Work out the finished part from the listing and answer in its coordinate system (mm). A direction names the side the tool comes from. Give positions to 0.01 mm unless a question says otherwise; leave off trailing zeros. Order: outer loops, then holes, each group sorted by start corner. A loop starts at its lowest first (then second) coordinate and runs counter-clockwise, first axis right, second up. Notation, with made-up numbers: (-30.75, 6) -> (-24.75, 6) arc R17 ccw to (-24.75, 15) -> close; hole circle Ø2 at (-39, 57.5). An arc over 180 degrees is marked (long way). Use a Markdown table: item, result. Add a question column.
```python
from build123d import *

# Parameters (mm, degrees)
EXTRUDE_1_DEPTH     = 18
CUT_EXTRUDE_1_DEPTH = 16
HOLE_WIZARD_M51_D   = 5.5
HOLE_WIZARD_M52_D   = 5.5


with BuildPart() as part:
    # Эскиз1 → Бобышка-Вытянуть1 (new body)
    with BuildSketch(Plane.XY):
        Polygon((0, 0), (0, 8), (30.5, 38.5), (38.5, 38.5), (38.5, 0), align=None)
    extrude(amount=EXTRUDE_1_DEPTH)

    # Эскиз2 → Вырез-Вытянуть1 (cut)
    with BuildSketch(Plane.XY.offset(18)):
        Polygon((0, 2), (36.5, 2), (36.5, 38.5), (30.5, 38.5), (0, 8), align=None)
    extrude(amount=-CUT_EXTRUDE_1_DEPTH, mode=Mode.SUBTRACT)

    # Отверстие с зазором M51 (through all)
    with Locations(Plane(origin=(0, 2, 0), x_dir=(1, 0, 0), z_dir=(0, 1, 0))):
        with Locations((8.5, -9), (28.5, -9)):
            Hole(HOLE_WIZARD_M51_D / 2)

    # Отверстие с зазором M52 (through all)
    with Locations(Plane.ZY.offset(-36.5)):
        with Locations((9, 10), (9, 30)):
            Hole(HOLE_WIZARD_M52_D / 2)


solid = part.part
```
1) The part is cut by section A-A, the plane y = 30. Determine the outline of the cut face in (x, z), then the cut area to 3 significant figures.
2) The part is cut by section D-D, the plane y = 16.5. Determine the outline of the cut face in (x, z), then the cut area to 3 significant figures.
3) Determine the mould class of faces 1 (the flat face through (15, 23, 1)), 2 (the cylindrical face through (37.51, 32.32, 7.52)), 3 (the flat face through (38.5, 20, 9)), 4 (the cylindrical face through (31.247, 0.986, 8.879)) for opening direction X: released by +X, released by -X, zero draft, split by the parting line, or undercut.
4) Straight lines are drawn through the part: line 1 (Y direction, x = 37, z = 9); line 2 (X direction, y = 1.4, z = 9); line 3 (Z direction, x = 8.5, y = 0.9). For each, find the intervals that lie inside material, in ascending order.
5) Which of the six approach directions +Z, -Z, +X, -X, +Y, -Y give full straight-line access (tool end or side, diameter ignored) to faces 5 (the cylindrical face through (37.51, 12.32, 7.52)), 6 (the flat face through (18, 2, 10))?
6) The part is cut by section C-C, the plane x = 28.5. Determine the outline of the cut face in (y, z), then the cut area to 3 significant figures.
7) The part is cut by section B-B, the plane z = 9. Determine the outline of the cut face in (x, y).
8) Flat-ended cylindrical pins translate along their axes: pin 1 (10 mm diameter, centred on x = 11.5, y = 10, fed in from +Z); pin 2 (1 mm diameter, centred on y = 34.5, z = 12, fed in from -X); pin 3 (5 mm diameter, centred on x = 28.5, z = 9, fed in from -Y); pin 4 (1.5 mm diameter, centred on x = 15.5, z = 4.5, fed in from +Y). Find the tip coordinate at first contact, or state that the pin passes through.
A:
| question | item | result |
|---|---|---|
| 1 | outline | (22, 0) -> (38.5, 0) -> (38.5, 6.25) -> (36.5, 6.25) -> (36.5, 2) -> (22, 2) -> close; (36.5, 11.75) -> (38.5, 11.75) -> (38.5, 18) -> (36.5, 18) -> close |
| 1 | area | 54.0 mm^2 |
| 2 | outline | (8.5, 0) -> (38.5, 0) -> (38.5, 18) -> (36.5, 18) -> (36.5, 2) -> (8.5, 2) -> close |
| 2 | area | 92.0 mm^2 |
| 3 | face 1 | released by -X |
| 3 | face 2 | zero draft |
| 3 | face 3 | released by +X |
| 3 | face 4 | undercut |
| 4 | line 1 | 0 to 7.25, 12.75 to 27.25, 32.75 to 38.5 |
| 4 | line 2 | 0 to 5.75, 11.25 to 25.75, 31.25 to 38.5 |
| 4 | line 3 | 0 to 6.25, 11.75 to 18 |
| 5 | face 5 | +X, -X |
| 5 | face 6 | +Z, -X, +Y |
| 6 | outline | (0, 0) -> (36.5, 0) -> (36.5, 2) -> (2, 2) -> (2, 6.25) -> (0, 6.25) -> close; (0, 11.75) -> (2, 11.75) -> (2, 18) -> (0, 18) -> close |
| 6 | area | 94.0 mm^2 |
| 7 | outline | (0, 0) -> (5.75, 0) -> (5.75, 2) -> (0, 2) -> close; (11.25, 0) -> (25.75, 0) -> (25.75, 2) -> (11.25, 2) -> close; (31.25, 0) -> (38.5, 0) -> (38.5, 7.25) -> (36.5, 7.25) -> (36.5, 2) -> (31.25, 2) -> close; (36.5, 12.75) -> (38.5, 12.75) -> (38.5, 27.25) -> (36.5, 27.25) -> close; (36.5, 32.75) -> (38.5, 32.75) -> (38.5, 38.5) -> (36.5, 38.5) -> close |
| 8 | pin 1 | z = 2 |
| 8 | pin 2 | x = 36.5 |
| 8 | pin 3 | through |
| 8 | pin 4 | y = 2 |
